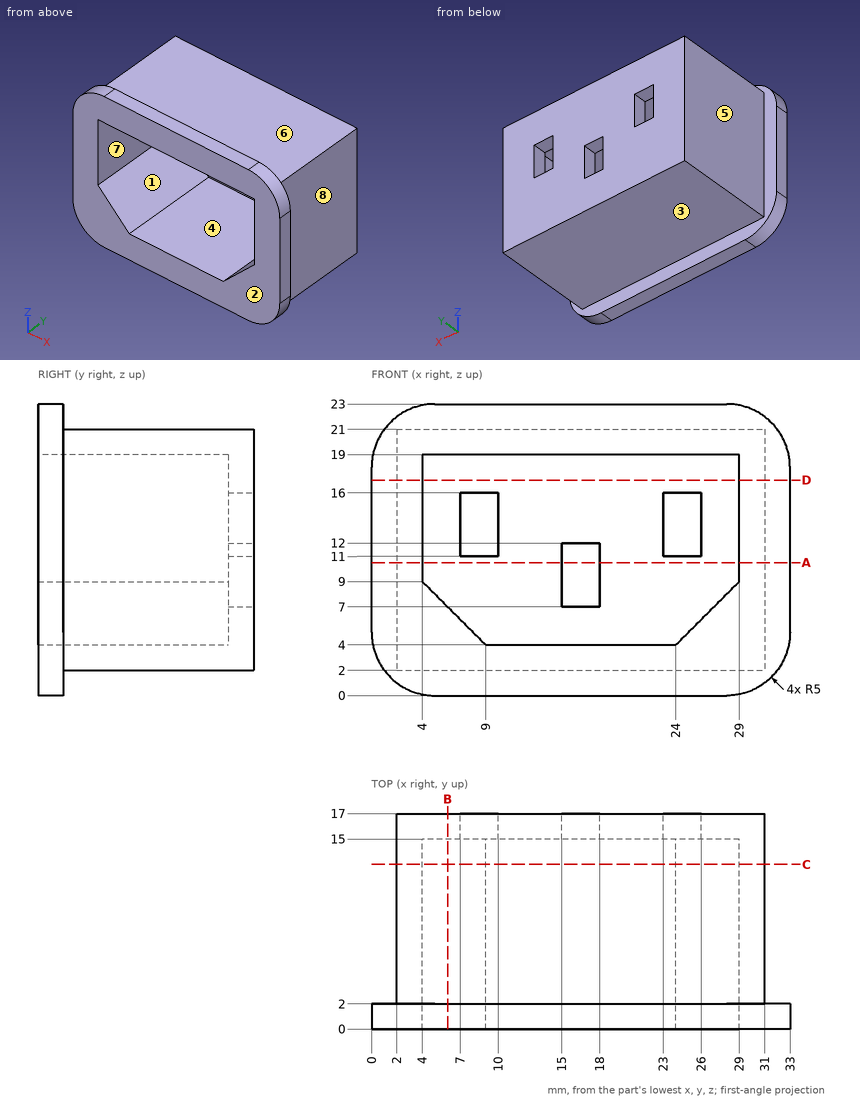
Here's the drawing with two shaded views (mm, measured from the low corner). I have some questions. A direction names the side the tool comes from. Coordinates: 2 decimals unless noted, no trailing zeros. Loops run counter-clockwise (first coordinate to the right, second up) from the corner with the lowest first, then second, coordinate; pieces in that order, holes last.
Item 1: Suppose I cut it at B-B (x = 6). Please give me the cut outline in (y, z).
Answers below:
outline: (0, 0) - (2, 0) - (2, 2) - (17, 2) - (17, 21) - (2, 21) - (2, 23) - (0, 23) - (0, 19) - (15, 19) - (15, 7) - (0, 7) - close
Item 2: Please list where these lines run through material, in increasing order: L1, parallel to X at y = 2.5, z = 6; L2, parallel to X at y = 8.5, z = 9.75; L3, parallel to X at y = 16, z = 11.25.
Answers below:
L1: x = 2 to 7, 26 to 31
L2: x = 2 to 4, 29 to 31
L3: x = 2 to 7, 10 to 15, 18 to 23, 26 to 31
Item 3: I'm going to push flat-ended pins straight in: pin 1 (0.6 mm diameter, centred on x = 16, y = 16, fed in from +Z); pin 2 (0.6 mm diameter, centred on x = 8, y = 16, fed in from -Z); pin 3 (1 mm diameter, centred on y = 9.5, z = 7.5, fed in from +X). Where does each tip first touch, or does it pass through?
Answers below:
pin 1: stops at z = 21
pin 2: stops at z = 2
pin 3: stops at x = 31
Item 4: Suppose I cut it at C-C (y = 13). Please give me the cut outline in (x, z), then the cut area to 3 significant figures.
Answers below:
outline: (2, 2) - (31, 2) - (31, 21) - (2, 21) - close; hole (4, 9) - (9, 4) - (24, 4) - (29, 9) - (29, 19) - (4, 19) - close
area: 201 mm2
Item 5: Suppose I cut it at D-D (z = 17). Please give me the cut outline in (x, y), then the cut area to 3 significant figures.
Answers below:
outline: (0, 0) - (4, 0) - (4, 15) - (29, 15) - (29, 0) - (33, 0) - (33, 2) - (31, 2) - (31, 17) - (2, 17) - (2, 2) - (0, 2) - close
area: 126 mm2
Item 6: Which directions (+Z, -Z, +X, -X, +Y, -Y) give clear straight access to the entire face, cutting with the end or side of a thin tool? Please do the marked faces 5, 6, 7 and 8.
Answers below:
face 5: +Z, -Z, -X, +Y
face 6: +Z, +X, -X, +Y
face 7: -Y
face 8: +Z, -Z, +X, +Y
Item 7: Suppose I cut it at A-A (z = 10.5). Please give me the cut outline in (x, y), then the cut area to 3 significant figures.
Answers below:
outline: (0, 0) - (4, 0) - (4, 15) - (15, 15) - (15, 17) - (2, 17) - (2, 2) - (0, 2) - close; (18, 15) - (29, 15) - (29, 0) - (33, 0) - (33, 2) - (31, 2) - (31, 17) - (18, 17) - close
area: 120 mm2
Item 8: If we mould it in two halves opening along Z, with no side actions, what happens to the marked faces 1, 2, 3 and 4? For each: released by +Z, released by -Z, zero draft, split by the parting line, or undercut.
Answers below:
face 1: undercut
face 2: zero draft
face 3: released by -Z
face 4: undercut
